Here's how the part is built. I have some questions about the finished solid (model axes, mm). Coordinates: 2 decimals unless noted, no trailing zeros. Write each loop counter-clockwise with the first axis right and the second up, starting at its lowest first coordinate (ties: lowest second). Pieces come first, ordered by that corner, then holes. Notation, with made-up numbers: (-37, -39.5) - (-6, -39.5) arc R19 ccw to (-6, -17.5) - close; hole circle Ø10 at (72.25, 73). An arc over 180 degrees is marked (long way). Answer in a Markdown table with one row per item. Add a question column.
Item 1: Imagine slicing it at B-B (y = -19). Please give me the cut outline in (x, z).
Item 2: If I drill on probe 1 along Z at (x, y) = (0, -19.5); probe 2 along Z at (x, y) = (15, -1.25); probe 3 along X at (y, z) = (-19, -12), over which ranges is the centre line in solid material (lowest first)? Write a range as from..to.
Item 3: Imagine slicing it at C-C (x = -31.5). Please give me the cut outline in (y, z).
Item 4: We'd pull the mould along Z, two halves only. Please class faces 1 (the face through (23.846, -12.325, 7.509)), 2 (the face through (37.5, -12, 247)), 3 (the face through (0.82, -12.32, 537.49)), 4 (the face through (-3.255, -12.325, 524.787)): +Z half, -Z half, draft (parallel to the pull), parting line (faces both ways), or undercut.
Item 5: Imagine slicing it at A-A (x = 0). Please give me the cut outline in (y, z), plus the area to 3 significant figures.
Item 6: I'm going to push flat-ended pins straight in: pin 1 (1 mm diameter, centred on x = 11.5, y = -21, fed in from -Z); pin 2 (4 mm diameter, centred on x = -7, y = -14.5, fed in from -Z); pin 3 (1.5 mm diameter, centred on x = -15, y = -4.5, fed in from +Z). Where does each tip first touch, or does it pass through?
from build123d import *

# Parameters (mm, degrees)
F0_R     = 25
F1_DEPTH = 25


with BuildPart() as f1:
    # F0 (on Front) → F1 (new body)
    with BuildSketch(Plane.XZ):
        with BuildLine():
            ThreePointArc((-37.5, 0), (0, -37.5), (37.5, 0))
            ThreePointArc((37.5, 0), (0, 37.5), (-37.5, 0))
        make_face()
        Circle(F0_R, mode=Mode.SUBTRACT)
        with BuildLine():
            ThreePointArc((-37.5, 500), (0, 462.5), (37.5, 500))
            ThreePointArc((37.5, 500), (0, 537.5), (-37.5, 500))
        make_face()
        with Locations((0, 500)):
            Circle(F0_R, mode=Mode.SUBTRACT)
        with BuildLine():
            ThreePointArc((-37.5, 0), (0, 37.5), (37.5, 0))
            Line((37.5, 0), (37.5, 500))
            ThreePointArc((37.5, 500), (0, 462.5), (-37.5, 500))
            Line((-37.5, 500), (-37.5, 0))
        make_face()
    extrude(amount=F1_DEPTH)


solid = f1.part
Here are the results:
| question | item | result |
|---|---|---|
| 1 | outline | (-37.5, 0) arc R37.5 ccw to (37.5, 0) - (37.5, 500) arc R37.5 ccw to (-37.5, 500) - close; hole circle Ø50 at (0, 0); hole circle Ø50 at (0, 500) |
| 2 | probe 1 | z = -37.5..-25, 25..475, 525..537.5 |
| 2 | probe 2 | z = -34.37..-20, 20..480, 520..534.37 |
| 2 | probe 3 | x = -35.53..-21.93, 21.93..35.53 |
| 3 | outline | (-25, -20.35) - (0, -20.35) - (0, 520.35) - (-25, 520.35) - close |
| 4 | face 1 | undercut |
| 4 | face 2 | draft |
| 4 | face 3 | +Z half |
| 4 | face 4 | undercut |
| 5 | outline | (-25, -37.5) - (0, -37.5) - (0, -25) - (-25, -25) - close; (-25, 25) - (0, 25) - (0, 475) - (-25, 475) - close; (-25, 525) - (0, 525) - (0, 537.5) - (-25, 537.5) - close |
| 5 | area | 11,900 mm2 |
| 6 | pin 1 | stops at z = -35.85 |
| 6 | pin 2 | stops at z = -37.17 |
| 6 | pin 3 | stops at z = 534.69 |
